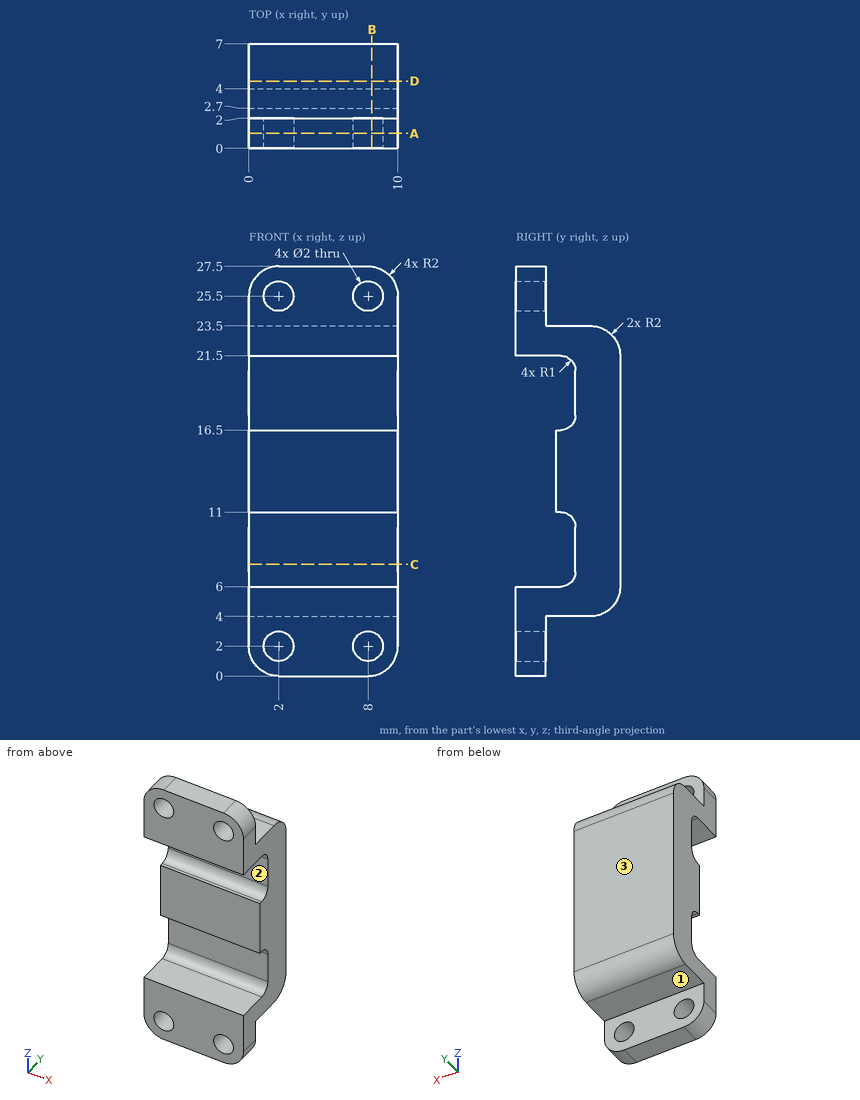
Answer from the drawing. Dimensions are ordinates in mm from the lowest x, y and z of the part. A direction names the side the tool comes from. Coordinates: 2 decimals unless noted, no trailing zeros. Order: outer loops, then holes, each group sorted by start corner. A loop starts at its lowest first (then second) coordinate and runs counter-clockwise, first axis right, second up. Notation, with made-up numbers: (-33.5, 83.25) - (-14.5, 83.25) arc R16 cw to (-14.5, 100.25) - close; hole circle Ø8 at (5.25, 25.25). An arc over 180 degrees is marked (long way). Answer as a JSON object with one key per item and string values. Group by question number.
Item 1: Section C-C (z = 7.5) is taken. Give the vertices of the cut face in (x, y).
Item 2: Section A-A (y = 1) is taken. Give the vertices of the cut face in (x, z).
Item 3: Section D-D (y = 4.5) is taken. Give the vertices of the cut face in (x, z).
Item 4: Flat-ended cylindrical pins translate along their axes: P1, Ø4, axis at x = 3.5, z = 3.5, coming from the +Y side; P2, Ø0.9, axis at x = 5, z = 8.5, coming from the -Y side; P3, Ø3.5, axis at x = 5, z = 19.5, coming from the -Y side; P4, Ø3, axis at x = 2, z = 25.5, coming from the -Y side. Find the tip coordinate at first contact, or state that the pin passes through.
Item 5: Consider probe 1 along Z at (x, y) = (8, 1.45); probe 2 along X at (y, z) = (1, 25.5); probe 3 along Z at (x, y) = (3.25, 3.25). Determine where each line is inside the solid, lowest interval first. Write a range as from..to.
Item 6: A tool of negligible diameter and unlimited length cuts with its end or side. For the marked faces 1, 2 and 3, from which of +Z, -Z, +X, -X, +Y, -Y can it reach the whole face along a straight path? Write none if from no direction.
Item 7: Section B-B (x = 8.25) is taken. State how many separate pieces and enclosed holes the cut face has, plus the area to 3 significant figures.
Results are:
{
 "1": {"outline": "(0, 4) - (10, 4) - (10, 7) - (0, 7) - close"},
 "2": {"outline": "(0, 2) arc R2 ccw to (2, 0) - (8, 0) arc R2 ccw to (10, 2) - (10, 6) - (0, 6) - close; (0, 21.5) - (10, 21.5) - (10, 25.5) arc R2 ccw to (8, 27.5) - (2, 27.5) arc R2 ccw to (0, 25.5) - close; hole circle Ø2 at (2, 2); hole circle Ø2 at (2, 25.5); hole circle Ø2 at (8, 2); hole circle Ø2 at (8, 25.5)"},
 "3": {"outline": "(0, 4) - (10, 4) - (10, 23.5) - (0, 23.5) - close"},
 "4": {"P1": "stops at y = 6.94", "P2": "stops at y = 4", "P3": "stops at y = 3.66", "P4": "stops at y = 0"},
 "5": {"probe 1": "z = 0..1, 3..6, 21.5..24.5, 26.5..27.5", "probe 2": "x = 0..1, 3..7, 9..10", "probe 3": "z = 4..6.03, 10.97..16.53, 21.47..23.5"},
 "6": {"face 1": "-Z, +X, -X, +Y", "face 2": "+X, -X, -Y", "face 3": "+Z, -Z, +X, -X, +Y"},
 "7": {"separate pieces": "3", "enclosed holes": "0", "area": "89.0 mm^2"}
}
